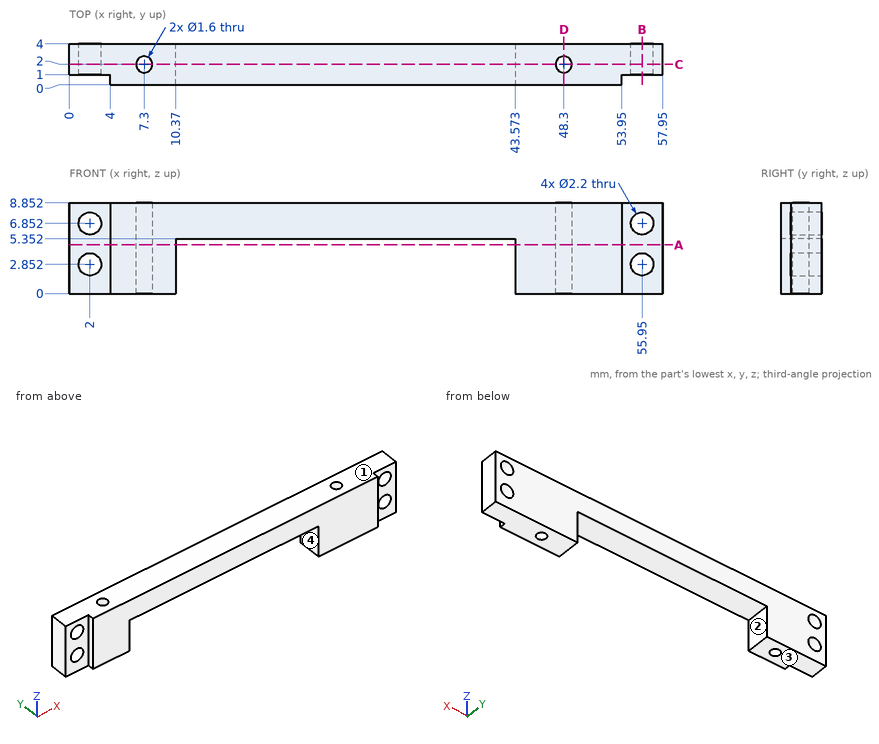
Design review of the part shown in the three views and the two pictorial views. Dimensions are in mm from the part's minimum x, y and z. A direction names the side the tool comes from. Round coordinates to 2 decimals unless told otherwise and drop trailing zeros. Write each loop counter-clockwise with the first axis right and the second up, starting at its lowest first coordinate (ties: lowest second). Pieces come first, ordered by that corner, then holes. Notation, with made-up numbers: (-14.75, -17.75) - (7.25, -17.75) arc R27 cw to (7.25, 15.25) - close; hole circle Ø9 at (67, 84). An arc over 180 degrees is marked (long way). Answer as CSV lines item,"result". Start each with the question number.
(1) Add section B-B, the plane x = 55.95. State the section outline as (y, z) points.
(2) Machinability: for the marked faces 1 and 2, which of the approach directions +Z, -Z, +X, -X, +Y, -Y give a long, thin tool a straight path to every point of the face, cutting with its end or side? Answer none if there is none.
(3) For pin 1 (1.2 mm diameter, centred on x = 57, z = 3, fed in from -Y); pin 2 (1 mm diameter, centred on x = 27.5, y = 0.5, fed in from -Z); pin 3 (0.5 mm diameter, centred on y = 0.5, z = 5, fed in from +X), all flat-tipped, find the tip position at first contact; note any pin that passes through.
(4) For line 1 (Z direction, x = 55.95, y = 3.1); line 2 (Y direction, x = 48.3, z = 3.5); line 3 (X direction, y = 0.95, z = 5.25), list the stretches that pass through material, from the lowest coordinate up.
(5) Add section C-C, the plane y = 2. State the section outline as (x, z) points.
(6) Add section A-A, the plane z = 4.75. State the section outline as (x, y) points, plus the area to 3 significant figures.
(7) Add section D-D, the plane x = 48.3. State the section outline as (y, z) points.
(8) Mouldability with a two-part tool opening along X and no side actions: class the marked faces 3 and 4 as +X half, -X half, draft (parallel to the pull), parting line (faces both ways), or undercut.
From the geometry:
1,outline,"(1, 0) - (4, 0) - (4, 1.75) - (1, 1.75) - close; (1, 3.95) - (4, 3.95) - (4, 5.75) - (1, 5.75) - close; (1, 7.95) - (4, 7.95) - (4, 8.85) - (1, 8.85) - close"
2,face 1,"+Z, +X, -X, +Y, -Y"
2,face 2,"-Z, +Y, -Y"
3,pin 1,"stops at y = 1"
3,pin 2,"stops at z = 5.35"
3,pin 3,"stops at x = 53.95"
4,line 1,"z = 0 to 1.75, 3.95 to 5.75, 7.95 to 8.85"
4,line 2,"y = 0 to 1.2, 2.8 to 4"
4,line 3,"x = 4 to 10.37, 43.57 to 53.95"
5,outline,"(0, 0) - (6.5, 0) - (6.5, 8.85) - (0, 8.85) - close; (8.1, 0) - (10.37, 0) - (10.37, 5.35) - (43.57, 5.35) - (43.57, 0) - (47.5, 0) - (47.5, 8.85) - (8.1, 8.85) - close; (49.1, 0) - (57.95, 0) - (57.95, 8.85) - (49.1, 8.85) - close; hole circle Ø2.2 at (2, 2.85); hole circle Ø2.2 at (2, 6.85); hole circle Ø2.2 at (55.95, 2.85); hole circle Ø2.2 at (55.95, 6.85)"
6,outline,"(0, 1) - (4, 1) - (4, 0) - (10.37, 0) - (10.37, 4) - (0, 4) - close; (43.57, 0) - (53.95, 0) - (53.95, 1) - (57.95, 1) - (57.95, 4) - (43.57, 4) - close; hole circle Ø1.6 at (7.3, 2); hole circle Ø1.6 at (48.3, 2)"
6,area,"87.0 mm²"
7,outline,"(0, 0) - (1.2, 0) - (1.2, 8.85) - (0, 8.85) - close; (2.8, 0) - (4, 0) - (4, 8.85) - (2.8, 8.85) - close"
8,face 3,"draft"
8,face 4,"undercut"
